from build123d import *

# Parameters (mm, degrees)
F1_DEPTH = 440
F3_DEPTH = 25.4


with BuildPart() as f1:
    # F0 (on Front) → F1 (new body, symmetric)
    with BuildSketch(Plane.XZ):
        Polygon((20.2946, 0), (20.2946, 20.3), (-14.7054, 20.3), (-14.7054, 13.3), (3, 13.3), (3, 10), (0, 10), (0, 0), align=None)
    extrude(amount=F1_DEPTH, both=True)

    # F2 (on face) → F3 (cut)
    with BuildSketch(Plane.XY.offset(20.3)):
        Polygon((-14.7054, 405), (20.2946, 440), (-14.7054, 440), align=None)
        Polygon((-14.7054, -440), (20.2946, -440), (-14.7054, -405), align=None)
    extrude(amount=-F3_DEPTH, mode=Mode.SUBTRACT)


solid = f1.part
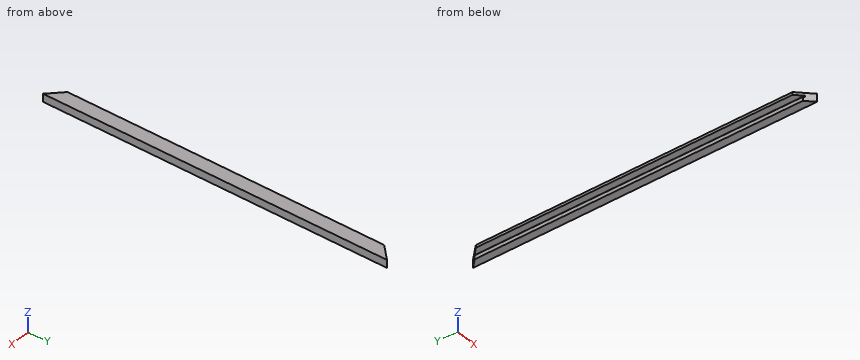
CAD build for the part. Positions are in the model's coordinates, mm. Coordinates: 2 decimals unless noted, no trailing zeros. Order: outer loops, then holes, each group sorted by start corner. A loop starts at its lowest first (then second) coordinate and runs counter-clockwise, first axis right, second up. Notation, with made-up numbers: (11.25, 79) -> (48.25, 79) arc R22 cw to (48.25, 106) -> close; hole circle Ø10 at (14.25, -14). An arc over 180 degrees is marked (long way). Answer in a Markdown table with one row per item.
1) Drill centre lines: line 1 (Z direction, x = -10, y = 136.5); line 2 (X direction, y = -79, z = 11.5); line 3 (Y direction, x = 3, z = 14.5). Where is each one in solid material? Low to high.
Check values:
| item | result |
|---|---|
| line 1 | 13.3 to 20.3 |
| line 2 | 3 to 20.29 |
| line 3 | -422.71 to 422.71 |
2) Band-saw the part on A-A (y = 0). List the corners of the cut face in (x, z).
Check values:
| item | result |
|---|---|
| outline | (-14.71, 13.3) -> (3, 13.3) -> (3, 10) -> (0, 10) -> (0, 0) -> (20.29, 0) -> (20.29, 20.3) -> (-14.71, 20.3) -> close |
3) Flat gauge pins, fed straight in: P1, Ø2, axis at x = 16.5, z = 8, coming from the +Y side; P2, Ø5, axis at y = 22.5, z = 3, coming from the -X side; P3, Ø3, axis at x = 7.5, z = 18, coming from the -Y side. Where does each tip first touch, or does it go through?
Check values:
| item | result |
|---|---|
| P1 | y = 437.21 |
| P2 | x = 0 |
| P3 | y = -428.71 |
4) Band-saw the part on C-C (x = 13). List the corners of the cut face in (y, z), and give its area (3 significant figures).
Check values:
| item | result |
|---|---|
| outline | (-432.71, 0) -> (432.71, 0) -> (432.71, 20.3) -> (-432.71, 20.3) -> close |
| area | 17,600 mm2 |
5) Band-saw the part on B-B (z = 3.5). List the corners of the cut face in (x, y), and give its area (3 significant figures).
Check values:
| item | result |
|---|---|
| outline | (0, -419.71) -> (20.29, -440) -> (20.29, 440) -> (0, 419.71) -> close |
| area | 17,400 mm2 |
